```python
from build123d import *

# Parameters (mm, degrees)
F0_R     = 8.9291855446
F0_W     = 1.8887050901
F0_H     = 16.251400295
F1_DEPTH = 5.08


with BuildPart() as f1:
    # F0 (on Top) → F1 (new body)
    with BuildSketch(Plane.XY):
        with BuildLine():
            Line((44.45, -11.43), (44.45, 11.43))
            Line((44.45, 11.43), (-44.45, 11.43))
            ThreePointArc((-44.45, 11.43), (-67.8202265578, 0), (-44.45, -11.43))
            Line((-44.45, -11.43), (44.45, -11.43))
        make_face()
        with BuildLine():
            Line((-19.3083044142, 0), (-23.491198197, -5.8829421178))
            Line((-23.491198197, -5.8829421178), (-27.6740919799, 0))
            ThreePointArc((-27.6740919799, 0), (-27.9666728456, 2.6362555137), (-25.8814226836, 4.2755170725))
            ThreePointArc((-25.8814226836, 4.2755170725), (-24.4455751804, 4.0138821459), (-23.491198197, 2.9096740764))
            ThreePointArc((-23.491198197, 2.9096740764), (-22.5368212136, 4.0138821459), (-21.1009737104, 4.2755170725))
            ThreePointArc((-21.1009737104, 4.2755170725), (-19.0157235484, 2.6362555137), (-19.3083044142, 0))
        make_face(mode=Mode.SUBTRACT)
        with BuildLine():
            add(Edge.make_bspline(
                [(-1.1741983702, 5.1239690358), (0.5040073817, 3.2998977303), (0.5040073817, -0.1196720545)],
                knots=[0, 0, 0, 1, 1, 1], degree=2))
            add(Edge.make_bspline(
                [(0.5040073817, -0.1196720545), (0.5040073817, -3.5332267649), (-1.1877322875, -5.366320682)],
                knots=[0, 0, 0, 1, 1, 1], degree=2))
            add(Edge.make_bspline(
                [(-1.1877322875, -5.366320682), (-2.8794719568, -7.1994145992), (-6.037386006, -7.1994145992)],
                knots=[0, 0, 0, 1, 1, 1], degree=2))
            add(Edge.make_bspline(
                [(-6.037386006, -7.1994145992), (-9.1953000553, -7.1994145992), (-10.8870397245, -5.366320682)],
                knots=[0, 0, 0, 1, 1, 1], degree=2))
            add(Edge.make_bspline(
                [(-10.8870397245, -5.366320682), (-12.5787793938, -3.5332267649), (-12.5787793938, -0.1016268314)],
                knots=[0, 0, 0, 1, 1, 1], degree=2))
            add(Edge.make_bspline(
                [(-12.5787793938, -0.1016268314), (-12.5787793938, 3.3299731022), (-10.8825284187, 5.1390067218)],
                knots=[0, 0, 0, 1, 1, 1], degree=2))
            add(Edge.make_bspline(
                [(-10.8825284187, 5.1390067218), (-9.1862774437, 6.9480403414), (-6.0193407829, 6.9480403414)],
                knots=[0, 0, 0, 1, 1, 1], degree=2))
            add(Edge.make_bspline(
                [(-6.0193407829, 6.9480403414), (-2.8524041221, 6.9480403414), (-1.1741983702, 5.1239690358)],
                knots=[0, 0, 0, 1, 1, 1], degree=2))
        make_face(mode=Mode.SUBTRACT)
        with BuildLine():
            Line((14.883042686, -7.0099397562), (11.7642266202, -7.0099397562))
            Line((11.7642266202, -7.0099397562), (10.9551991161, -3.3347293104))
            Line((10.9551991161, -3.3347293104), (9.8664706534, 1.3089081106))
            Line((9.8664706534, 1.3089081106), (9.8003048353, 1.3089081106))
            Line((9.8003048353, 1.3089081106), (7.8814961082, -7.0099397562))
            Line((7.8814961082, -7.0099397562), (4.7987704887, -7.0099397562))
            Line((4.7987704887, -7.0099397562), (1.8122860592, 3.4983951848))
            Line((1.8122860592, 3.4983951848), (4.6694463895, 3.4983951848))
            Line((4.6694463895, 3.4983951848), (5.881483877, -1.1542648478))
            add(Edge.make_bspline(
                [(5.881483877, -1.1542648478), (6.1732149844, -2.4054003187), (6.4739687034, -4.6039100044)],
                knots=[0, 0, 0, 1, 1, 1], degree=2))
            Line((6.4739687034, -4.6039100044), (6.5281043728, -4.6039100044))
            add(Edge.make_bspline(
                [(6.5281043728, -4.6039100044), (6.5672023563, -3.8881161533), (6.8589334637, -2.3392345005)],
                knots=[0, 0, 0, 1, 1, 1], degree=2))
            Line((6.8589334637, -2.3392345005), (7.0093103232, -1.5392296081))
            Line((7.0093103232, -1.5392296081), (8.3055588519, 3.4983951848))
            Line((8.3055588519, 3.4983951848), (11.4634729012, 3.4983951848))
            Line((11.4634729012, 3.4983951848), (12.6935556118, -1.5392296081))
            add(Edge.make_bspline(
                [(12.6935556118, -1.5392296081), (12.7326535953, -1.7467496742), (12.8123533308, -2.1512634262)],
                knots=[0, 0, 0, 1, 1, 1], degree=2))
            add(Edge.make_bspline(
                [(12.8123533308, -2.1512634262), (12.8920530663, -2.5557771782), (12.9672414961, -3.0114190625)],
                knots=[0, 0, 0, 1, 1, 1], degree=2))
            add(Edge.make_bspline(
                [(12.9672414961, -3.0114190625), (13.0424299258, -3.4670609467), (13.1040844382, -3.9031538392)],
                knots=[0, 0, 0, 1, 1, 1], degree=2))
            add(Edge.make_bspline(
                [(13.1040844382, -3.9031538392), (13.1657389506, -4.3392467317), (13.1747615622, -4.6039100044)],
                knots=[0, 0, 0, 1, 1, 1], degree=2))
            Line((13.1747615622, -4.6039100044), (13.2288972316, -4.6039100044))
            add(Edge.make_bspline(
                [(13.2288972316, -4.6039100044), (13.3161158101, -3.9272141367), (13.5311547192, -2.7482595584)],
                knots=[0, 0, 0, 1, 1, 1], degree=2))
            add(Edge.make_bspline(
                [(13.5311547192, -2.7482595584), (13.7461936282, -1.56930498), (13.8424348183, -1.1542648478)],
                knots=[0, 0, 0, 1, 1, 1], degree=2))
            Line((13.8424348183, -1.1542648478), (15.0995853636, 3.4983951848))
            Line((15.0995853636, 3.4983951848), (17.911632636, 3.4983951848))
            Line((17.911632636, 3.4983951848), (14.883042686, -7.0099397562))
        make_face(mode=Mode.SUBTRACT)
        with BuildLine():
            add(Edge.make_bspline(
                [(26.4440156434, -7.0159548306), (25.5898750815, -7.1994145992), (24.3567848337, -7.1994145992)],
                knots=[0, 0, 0, 1, 1, 1], degree=2))
            add(Edge.make_bspline(
                [(24.3567848337, -7.1994145992), (21.8214309827, -7.1994145992), (20.3928508176, -5.7979022688)],
                knots=[0, 0, 0, 1, 1, 1], degree=2))
            add(Edge.make_bspline(
                [(20.3928508176, -5.7979022688), (18.9642706525, -4.3963899383), (18.9642706525, -1.8309607155)],
                knots=[0, 0, 0, 1, 1, 1], degree=2))
            add(Edge.make_bspline(
                [(18.9642706525, -1.8309607155), (18.9642706525, 0.8096569371), (20.2845794788, 2.2517710196)],
                knots=[0, 0, 0, 1, 1, 1], degree=2))
            add(Edge.make_bspline(
                [(20.2845794788, 2.2517710196), (21.6048883051, 3.6938851021), (23.9357296271, 3.6938851021)],
                knots=[0, 0, 0, 1, 1, 1], degree=2))
            add(Edge.make_bspline(
                [(23.9357296271, 3.6938851021), (26.1613071476, 3.6938851021), (27.4019162383, 2.4262081766)],
                knots=[0, 0, 0, 1, 1, 1], degree=2))
            add(Edge.make_bspline(
                [(27.4019162383, 2.4262081766), (28.6425253291, 1.1585312511), (28.6425253291, -1.079076418)],
                knots=[0, 0, 0, 1, 1, 1], degree=2))
            Line((28.6425253291, -1.079076418), (28.6425253291, -2.4715661369))
            Line((28.6425253291, -2.4715661369), (21.8665440406, -2.4715661369))
            add(Edge.make_bspline(
                [(21.8665440406, -2.4715661369), (21.9146646356, -3.6926262359), (22.5913605033, -4.3783447152)],
                knots=[0, 0, 0, 1, 1, 1], degree=2))
            add(Edge.make_bspline(
                [(22.5913605033, -4.3783447152), (23.268056371, -5.0640631945), (24.48911647, -5.0640631945)],
                knots=[0, 0, 0, 1, 1, 1], degree=2))
            add(Edge.make_bspline(
                [(24.48911647, -5.0640631945), (25.439498222, -5.0640631945), (26.2846161723, -4.8670695085)],
                knots=[0, 0, 0, 1, 1, 1], degree=2))
            add(Edge.make_bspline(
                [(26.2846161723, -4.8670695085), (27.1297341227, -4.6700758226), (28.0500405027, -4.2369904673)],
                knots=[0, 0, 0, 1, 1, 1], degree=2))
            Line((28.0500405027, -4.2369904673), (28.0500405027, -6.4565529133))
            add(Edge.make_bspline(
                [(28.0500405027, -6.4565529133), (27.2981562053, -6.832495062), (26.4440156434, -7.0159548306)],
                knots=[0, 0, 0, 1, 1, 1], degree=2))
        make_face(mode=Mode.SUBTRACT)
        with BuildLine():
            Line((40.6726740882, -0.158770038), (40.6726740882, -7.0099397562))
            Line((40.6726740882, -7.0099397562), (37.8064911463, -7.0099397562))
            Line((37.8064911463, -7.0099397562), (37.8064911463, -0.8715563519))
            add(Edge.make_bspline(
                [(37.8064911463, -0.8715563519), (37.8064911463, 0.2652927058), (37.4019773943, 0.8337172347)],
                knots=[0, 0, 0, 1, 1, 1], degree=2))
            add(Edge.make_bspline(
                [(37.4019773943, 0.8337172347), (36.9974636423, 1.4021417635), (36.1132477085, 1.4021417635)],
                knots=[0, 0, 0, 1, 1, 1], degree=2))
            add(Edge.make_bspline(
                [(36.1132477085, 1.4021417635), (34.9102328326, 1.4021417635), (34.3748912128, 0.5991293339)],
                knots=[0, 0, 0, 1, 1, 1], degree=2))
            add(Edge.make_bspline(
                [(34.3748912128, 0.5991293339), (33.839549593, -0.2038830958), (33.839549593, -2.0655486163)],
                knots=[0, 0, 0, 1, 1, 1], degree=2))
            Line((33.839549593, -2.0655486163), (33.839549593, -7.0099397562))
            Line((33.839549593, -7.0099397562), (30.9733666512, -7.0099397562))
            Line((30.9733666512, -7.0099397562), (30.9733666512, 3.4983951848))
            Line((30.9733666512, 3.4983951848), (33.1628537253, 3.4983951848))
            Line((33.1628537253, 3.4983951848), (33.5478184856, 2.154026061))
            Line((33.5478184856, 2.154026061), (33.7072179567, 2.154026061))
            add(Edge.make_bspline(
                [(33.7072179567, 2.154026061), (34.188423907, 2.91493297), (35.0290305516, 3.304409036)],
                knots=[0, 0, 0, 1, 1, 1], degree=2))
            add(Edge.make_bspline(
                [(35.0290305516, 3.304409036), (35.8696371961, 3.6938851021), (36.9403204357, 3.6938851021)],
                knots=[0, 0, 0, 1, 1, 1], degree=2))
            add(Edge.make_bspline(
                [(36.9403204357, 3.6938851021), (38.7749181214, 3.6938851021), (39.7237961048, 2.7029015981)],
                knots=[0, 0, 0, 1, 1, 1], degree=2))
            add(Edge.make_bspline(
                [(39.7237961048, 2.7029015981), (40.6726740882, 1.7119180941), (40.6726740882, -0.158770038)],
                knots=[0, 0, 0, 1, 1, 1], degree=2))
        make_face(mode=Mode.SUBTRACT)
        with Locations((-53.3399991691, 0)):
            Circle(F0_R, mode=Mode.SUBTRACT)
        with Locations((-33.3491009139, 0.1086286247)):
            Rectangle(F0_W, F0_H, mode=Mode.SUBTRACT)
    extrude(amount=F1_DEPTH)


solid = f1.part
```
Model file for the job. Use its own axes, mm. A direction names the side the tool comes from. Give positions to 0.01 mm unless a question says otherwise; leave off trailing zeros. Write each loop counter-clockwise with the first axis right and the second up, starting at its lowest first coordinate (ties: lowest second). Pieces come first, ordered by that corner, then holes. Notation, with made-up numbers: (34.25, 85.25) -> (83.25, 85.25) arc R25 ccw to (83.25, 109.25) -> close; hole circle Ø6 at (26.5, -12.5). An arc over 180 degrees is marked (long way). Use CSV: the item, a comma, the result in double quotes. Start each with the question number.
1) Cut at A-A on x = -53.34. List the corners of the cut face in (y, z).
2) Cut at C-C on x = -24.5. List the corners of the cut face in (y, z).
3) Tool access for faces 1 (the flat face through (-12.5, 3.4, 5.08)), 2 (the cylindrical face through (-24.46, 4.02, 2.5)): list every direction of +Z, -Z, +X, -X, +Y, -Y with a clear straight run to the whole face (end or side of a thin tool).
4) Cut at D-D on y = 12.5. List the corners of the cut face in (x, z), plus the area to 3 significant figures.
5) Pin check, flat tips, straight feed: P1, Ø1.5, axis at x = 6, z = 3.5, coming from the +Y side; P2, Ø2, axis at x = 16.5, z = 2.5, coming from the -Y side; P3, Ø2, axis at x = -46, z = 0.5, coming from the +Y side. Stop position of each tip, or through.
6) Drill centre lines: L1, parallel to Y at x = -53.34, z = 3.75; L2, parallel to Y at x = 26.5, z = 3.8; L3, parallel to Y at x = -17, z = 3.8. Where is each one in solid material? Low to high.
7) Cut at B-B on z = 1.3. Count the separate pieces of the cut face and the enclosed holes in it, plus the area to 3 significant figures.
8) Two-plate mould, pull along Y, no slides. Class faces 3 (the flat face through (13, -7.01, 3)), 4 (the flat face through (-33, -8.017, 3)), 5 (the flat face through (-12.5, 3.4, 0)): released by +Y, released by -Y, zero draft, split by the parting line, or undercut.
Final values:
1,outline,"(-14.48, 0) -> (-8.93, 0) -> (-8.93, 5.08) -> (-14.48, 5.08) -> close; (8.93, 0) -> (14.48, 0) -> (14.48, 5.08) -> (8.93, 5.08) -> close"
2,outline,"(-11.43, 0) -> (-4.46, 0) -> (-4.46, 5.08) -> (-11.43, 5.08) -> close; (4.04, 0) -> (11.43, 0) -> (11.43, 5.08) -> (4.04, 5.08) -> close"
3,face 1,"+Z, +X, -X, +Y, -Y"
3,face 2,"+Z, -Z"
4,outline,"(-60.65, 0) -> (-46.03, 0) -> (-46.03, 5.08) -> (-60.65, 5.08) -> close"
4,area,"74.3 mm2"
5,P1,"stops at y = 11.43"
5,P2,"stops at y = -11.43"
5,P3,"stops at y = 13.02"
6,L1,"y = -14.48 to -8.93, 8.93 to 14.48"
6,L2,"y = -11.43 to -7, -4.81 to -2.47, 3.11 to 11.43"
6,L3,"y = -11.43 to 11.43"
7,separate pieces,"1"
7,enclosed holes,"7"
7,area,"1,870 mm2"
8,face 3,"undercut"
8,face 4,"undercut"
8,face 5,"zero draft"
